from build123d import *

# Parameters (mm, degrees)
AUFSATZ_LINEAR_AUSTRAGEN1_DEPTH = 15
AUFSATZ_LINEAR_AUSTRAGEN2_DEPTH = 150
SCHNITT_LINEAR_AUSTRAGEN1_REACH = 192.434
SCHNITT_LINEAR_AUSTRAGEN2_REACH = 190.733
SKIZZE4_R                       = 1.7
SKIZZE5_R                       = 3.25
SCHNITT_LINEAR_AUSTRAGEN3_DEPTH = 9
SCHNITT_LINEAR_AUSTRAGEN4_REACH = 201.985


with BuildPart() as part:
    # Skizze1 → Aufsatz-Linear austragen1 (new body)
    with BuildSketch(Plane.XY):
        Polygon((10, 0), (65.364729758, 0), (97, -9), (112, -9), (112, -24), (76.635270242, -24), (45, -15), (10, -15), align=None)
    extrude(amount=AUFSATZ_LINEAR_AUSTRAGEN1_DEPTH)

    # Skizze2 → Aufsatz-Linear austragen2 (add)
    with BuildSketch(Plane.XY.offset(15)):
        Polygon((112, -9), (112, -24), (97, -24), (97, -23), (99, -22), (102, -22), (102, -9), align=None)
    extrude(amount=AUFSATZ_LINEAR_AUSTRAGEN2_DEPTH)

    # Skizze3 → Schnitt-Linear austragen1 (cut, up to next)
    with BuildSketch(Plane.ZY.offset(-102), mode=Mode.PRIVATE) as schnitt_linear_austragen1_sk1:
        Polygon((165, -19), (45, -9), (165, -9), align=None)
    schnitt_linear_austragen1_tool1 = extrude(schnitt_linear_austragen1_sk1.sketch, amount=-SCHNITT_LINEAR_AUSTRAGEN1_REACH, mode=Mode.PRIVATE) & part.part
    add(schnitt_linear_austragen1_tool1.solids().sort_by_distance((102, -12.333333, 125))[0], mode=Mode.SUBTRACT)

    # Skizze4 → Schnitt-Linear austragen2 (cut, up to next)
    with BuildSketch(Plane.XY.offset(15), mode=Mode.PRIVATE) as schnitt_linear_austragen2_sk1:
        with Locations((36, -5)):
            Circle(SKIZZE4_R)
    schnitt_linear_austragen2_tool1 = extrude(schnitt_linear_austragen2_sk1.sketch, amount=-SCHNITT_LINEAR_AUSTRAGEN2_REACH, mode=Mode.PRIVATE) & part.part
    # Skizze4 → Schnitt-Linear austragen2 (cut, up to next)
    with BuildSketch(Plane.XY.offset(15), mode=Mode.PRIVATE) as schnitt_linear_austragen2_sk2:
        with Locations((27, -5)):
            Circle(SKIZZE4_R)
    schnitt_linear_austragen2_tool2 = extrude(schnitt_linear_austragen2_sk2.sketch, amount=-SCHNITT_LINEAR_AUSTRAGEN2_REACH, mode=Mode.PRIVATE) & part.part
    # Skizze4 → Schnitt-Linear austragen2 (cut, up to next)
    with BuildSketch(Plane.XY.offset(15), mode=Mode.PRIVATE) as schnitt_linear_austragen2_sk3:
        with Locations((18, -5)):
            Circle(SKIZZE4_R)
    schnitt_linear_austragen2_tool3 = extrude(schnitt_linear_austragen2_sk3.sketch, amount=-SCHNITT_LINEAR_AUSTRAGEN2_REACH, mode=Mode.PRIVATE) & part.part
    add(schnitt_linear_austragen2_tool1.solids().sort_by_distance((36, -5, 15))[0], mode=Mode.SUBTRACT)
    add(schnitt_linear_austragen2_tool2.solids().sort_by_distance((27, -5, 15))[0], mode=Mode.SUBTRACT)
    add(schnitt_linear_austragen2_tool3.solids().sort_by_distance((18, -5, 15))[0], mode=Mode.SUBTRACT)

    # Skizze5 → Schnitt-Linear austragen3 (cut)
    with BuildSketch(Plane.XY.offset(15)):
        with Locations((18, -5)):
            Circle(SKIZZE5_R)
        with Locations((27, -5)):
            Circle(SKIZZE5_R)
        with Locations((36, -5)):
            Circle(SKIZZE5_R)
    extrude(amount=-SCHNITT_LINEAR_AUSTRAGEN3_DEPTH, mode=Mode.SUBTRACT)

    # Skizze6 → Schnitt-Linear austragen4 (cut, up to next)
    with BuildSketch(Plane(origin=(0, -9, 0), x_dir=(1, 0, 0), z_dir=(0, 1, 0)), mode=Mode.PRIVATE) as schnitt_linear_austragen4_sk1:
        Polygon((112, -165), (107, -165), (112, -45), align=None)
    schnitt_linear_austragen4_tool1 = extrude(schnitt_linear_austragen4_sk1.sketch, amount=-SCHNITT_LINEAR_AUSTRAGEN4_REACH, mode=Mode.PRIVATE) & part.part
    add(schnitt_linear_austragen4_tool1.solids().sort_by_distance((110.333333, -9, 125))[0], mode=Mode.SUBTRACT)


solid = part.part
The listing builds one solid part. Answer for the finished solid, in the listing's coordinates (mm). A direction names the side the tool comes from. Give positions to 0.01 mm unless a question says otherwise; leave off trailing zeros. Write each loop counter-clockwise with the first axis right and the second up, starting at its lowest first coordinate (ties: lowest second). Pieces come first, ordered by that corner, then holes.
1) A tool of negligible diameter and unlimited length cuts with its end or side. For faces 1 (the face through (102, -24, 63)), 2 (the face through (39.002, -6.245, 10.563)), from which of +Z, -Z, +X, -X, +Y, -Y can it reach the whole face along a straight path? Write none if from no direction.
2) For a pull along Y with two mould halves and no side action, classify faces 3 (the face through (28, -15, 7)), 4 (the face through (34.65, -6.03, 3.04)), 5 (the face through (14.753, -4.857, 10.563)), 6 (the face through (100, -22, 89)) as pulls with the +Y half, pulls with the -Y half, needs draft (parallel to the pull), parting line crosses it, or undercut.
3) Section D-D (x = 94) is taken. Write down the section's boundary in (y, z), and give its area (3 significant figures).
4) Given P1, Ø4, axis at y = -18, z = 96.5, coming from the -X side; P2, Ø10, axis at x = 32, y = -9, coming from the +Z side; P3, Ø16.5, axis at x = 20.5, z = 7, coming from the -Y side, each flat-ended and moving along its own axis, determine where each tip first touches the part or whether it passes through.
5) Section C-C (z = 123) is taken. Write down the section's boundary in (x, y), and give its area (3 significant figures).
6) Section A-A (x = 36) is taken. Write down the section's boundary in (y, z), and give its area (3 significant figures).
7) Find the intervals of material crossed by L1, parallel to Y at x = 18, z = 3; L2, parallel to Y at x = 27, z = 10.25; L3, parallel to Z at x = 61, y = -10.75, in increasing order.
8) Section B-B (z = 24.5) is taken. Write down the section's boundary in (x, y), and give its area (3 significant figures).
Response:
1. face 1: +Z, -Z, +X, -X, -Y
1. face 2: +Z
2. face 3: pulls with the -Y half
2. face 4: undercut
2. face 5: undercut
2. face 6: pulls with the +Y half
3. outline: (-24, 0) - (-8.15, 0) - (-8.15, 15) - (-24, 15) - close
3. area: 238 mm2
4. P1: stops at x = 102
4. P2: stops at z = 15
4. P3: stops at y = -15
5. outline: (97, -24) - (108.75, -24) - (108.75, -15.5) - (102, -15.5) - (102, -22) - (99, -22) - (97, -23) - close
5. area: 66.4 mm2
6. outline: (-15, 0) - (-6.7, 0) - (-6.7, 6) - (-8.25, 6) - (-8.25, 15) - (-15, 15) - close; (-3.3, 0) - (0, 0) - (0, 15) - (-1.75, 15) - (-1.75, 6) - (-3.3, 6) - close
6. area: 146 mm2
7. L1: y = -15 to -6.7, -3.3 to 0
7. L2: y = -15 to -8.25, -1.75 to 0
7. L3: z = 0 to 15
8. outline: (97, -24) - (112, -24) - (112, -9) - (102, -9) - (102, -22) - (99, -22) - (97, -23) - close
8. area: 159 mm2
